```python
from build123d import *

# Parameters (mm, degrees)
F0_R     = 6.985
F1_DEPTH = 3.175
F2_R     = 2.38125
F3_DEPTH = 34.9758
F4_R     = 1.5748
F5_DEPTH = 7.112


with BuildPart() as f1:
    # F0 (on Top) → F1 (new body)
    with BuildSketch(Plane.XY):
        Circle(F0_R)
    extrude(amount=F1_DEPTH)

    # F2 (on face) → F3 (join)
    with BuildSketch(Plane.XY):
        Circle(F2_R)
    extrude(amount=-F3_DEPTH)

    # F4 (on face) → F5 (join)
    with BuildSketch(Plane.XY.offset(3.175)):
        with Locations((0, 4.826)):
            Circle(F4_R)
    extrude(amount=F5_DEPTH)


solid = f1.part
```
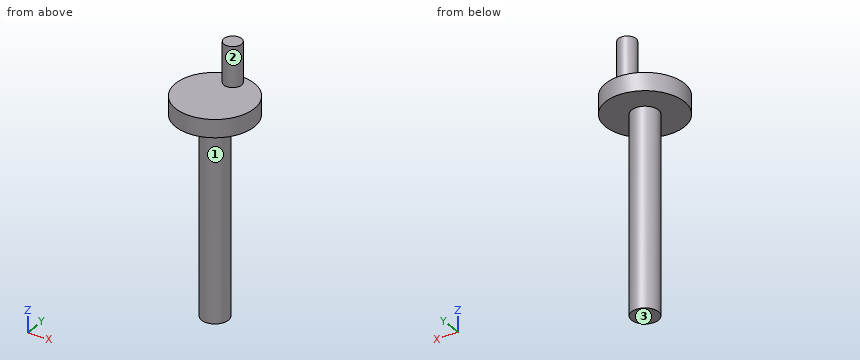
The listing builds one solid part. Answer for the finished solid, in the listing's coordinates (mm). Face numbers are marked on the shaded views. A direction names the side the tool comes from. Give positions to 0.01 mm unless a question says otherwise; leave off trailing zeros. Loops run counter-clockwise (first coordinate to the right, second up) from the corner with the lowest first, then second, coordinate; pieces in that order, holes last. Notation, with made-up numbers: (25, -31.75) - (66, -31.75) arc R11 cw to (66, -24.75) - close; hole circle Ø9 at (12, 4). An arc over 180 degrees is marked (long way). Return JSON: item names as keys, results as strings. Group by question number.
1. Which of the six approach directions +Z, -Z, +X, -X, +Y, -Y give full straight-line access (tool end or side, diameter ignored) to the marked faces 1, 2 and 3?
2. Find section D-D (y = -3.75). Write down the section's boundary in (x, z) (3 decimals).
3. Find section C-C (z = -14.5). Write down the section's boundary in (x, y).
4. Find section B-B (x = 0). Write down the section's boundary in (y, z) (3 decimals), then the cut area to 3 significant figures.
5. Find section A-A (y = 0). Write down the section's boundary in (x, z) (3 decimals), then the cut area to 3 significant figures.
6. Straight lines are drawn through the part: line 1 (Z direction, x = 3, y = 3) (3 decimals); line 2 (Z direction, x = 0.25, y = 1) (3 decimals); line 3 (Y direction, x = -2, z = -5). For each, find the intervals that lie inside material, in ascending order. Write a range as [from, to].
7. Given pin 1 Ø3 at (x, y) = (1, -5.5) entering from -Z; pin 2 Ø7 at (x, y) = (2, 1) entering from +Z; pin 3 Ø2 at (y, z) = (4.5, -6) entering from +X; pin 4 Ø6 at (x, z) = (5, -27) entering from -Y, each flat-ended and moving along its own axis, determine where each tip first touches the part or whether it passes through.
Verdict:
{
 "1": {"face 1": "-Z", "face 2": "+Z", "face 3": "-Z, +X, -X, +Y, -Y"},
 "2": {"outline": "(-5.893, 0) - (5.893, 0) - (5.893, 3.175) - (-5.893, 3.175) - close"},
 "3": {"outline": "circle Ø4.76 at (0, 0)"},
 "4": {"outline": "(-6.985, 0) - (-2.381, 0) - (-2.381, -34.976) - (2.381, -34.976) - (2.381, 0) - (6.985, 0) - (6.985, 3.175) - (6.401, 3.175) - (6.401, 10.287) - (3.251, 10.287) - (3.251, 3.175) - (-6.985, 3.175) - close", "area": "233 mm^2"},
 "5": {"outline": "(-6.985, 0) - (-2.381, 0) - (-2.381, -34.976) - (2.381, -34.976) - (2.381, 0) - (6.985, 0) - (6.985, 3.175) - (-6.985, 3.175) - close", "area": "211 mm^2"},
 "6": {"line 1": "z = [0, 3.175]", "line 2": "z = [-34.976, 3.175]", "line 3": "y = [-1.29, 1.29]"},
 "7": {"pin 1": "stops at z = 0", "pin 2": "stops at z = 10.29", "pin 3": "passes through", "pin 4": "stops at y = -1.29"}
}
